Verification items for the finished model (mm, model axes). Round coordinates to 2 decimals unless told otherwise and drop trailing zeros. Loops run counter-clockwise (first coordinate to the right, second up) from the corner with the lowest first, then second, coordinate; pieces in that order, holes last. Notation, with made-up numbers: M -37,60 L -18,60 A29 ccw -18,83 Z; hole C -37,51.25 d2. An arc over 180 degrees is marked long. Answer as CSV lines item,"result".
```python
from build123d import *

# Parameters (mm, degrees)
F0_W     = 53.34
F0_H     = 53.34
F1_DEPTH = 27.78125
F3_R     = 6.35
F4_DEPTH = 38.1
F5_SIZE  = 16.4973
F6_SIZE  = 16.51


with BuildPart() as f1:
    # F0 (on Front) → F1 (new body)
    with BuildSketch(Plane.XZ):
        Rectangle(F0_W, F0_H)
        with BuildLine():
            ThreePointArc((0, 25.4), (17.9605122421, 17.9605122421), (25.4, 0))
            ThreePointArc((25.4, 0), (17.9605122421, -17.9605122421), (0, -25.4))
            ThreePointArc((0, -25.4), (-25.4, 0), (0, 25.4))
        make_face(mode=Mode.SUBTRACT)
        with BuildLine():
            Line((0, -25.4), (0, 25.4))
            ThreePointArc((0, 25.4), (-25.4, 0), (0, -25.4))
        make_face()
        with BuildLine():
            ThreePointArc((0, -25.4), (17.9605122421, -17.9605122421), (25.4, 0))
            ThreePointArc((25.4, 0), (17.9605122421, 17.9605122421), (0, 25.4))
            Line((0, 25.4), (0, -25.4))
        make_face()
    extrude(amount=-F1_DEPTH)

    # F0 (on Front) → F2 (revolve, cut)
    with BuildSketch(Plane.XZ):
        with BuildLine():
            ThreePointArc((0, -25.4), (17.9605122421, -17.9605122421), (25.4, 0))
            ThreePointArc((25.4, 0), (17.9605122421, 17.9605122421), (0, 25.4))
            Line((0, 25.4), (0, -25.4))
        make_face()
    revolve(axis=Axis((0, 0, 0), (0, 0, 1)), mode=Mode.SUBTRACT)

    # F3 (on Top) → F4 (cut)
    with BuildSketch(Plane.XY):
        Circle(F3_R)
    extrude(amount=-F4_DEPTH, mode=Mode.SUBTRACT)

    # F5
    f5_edges = [f1.edges().sort_by_distance(p)[0] for p in [
        (26.67, 27.78125, 0),
    ]]
    chamfer(f5_edges, length=F5_SIZE)

    # F6
    f6_edges = [f1.edges().sort_by_distance(p)[0] for p in [
        (-26.67, 27.78125, 0),
    ]]
    chamfer(f6_edges, length=F6_SIZE)


solid = f1.part
```
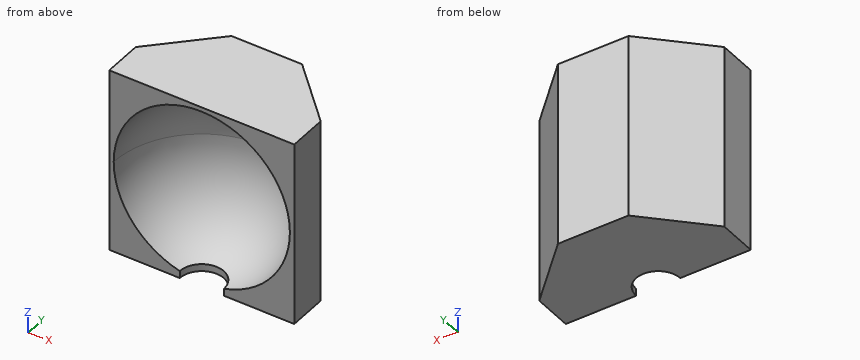
1) Go/stop test with a flat-tipped pin: pin 1 (8 mm diameter, centred on y = 22, z = 10.5, fed in from +X). Record where the tip stops, or that it passes through.
Here are the results:
pin 1,"stops at x = 19.95"
2) Section check B-B (y = 21). Record the cut outline in (x, z), plus the area to 3 significant figures.
Here are the results:
outline,"M -16.94,-26.67 L 16.95,-26.67 L 16.95,26.67 L -16.94,26.67 Z; hole C 0,0 d28.58"
area,"1,170 mm^2"
3) Section check D-D (y = 3.75). Record the cut outline in (x, z), plus the area to 3 significant figures.
Here are the results:
outline,"M -26.67,-26.67 L -5.12,-26.67 L -5.12,-24.59 A25.12 cw long 5.12,-24.59 L 5.12,-26.67 L 26.67,-26.67 L 26.67,26.67 L -26.67,26.67 Z"
area,"845 mm^2"
4) Section check C-C (z = 17). Record the cut outline in (x, y), plus the area to 3 significant figures.
Here are the results:
outline,"M -26.67,0 L -18.87,0 A18.87 cw 18.87,0 L 26.67,0 L 26.67,11.28 L 10.17,27.78 L -10.16,27.78 L -26.67,11.27 Z"
area,"650 mm^2"
5) Material ranges on probe 1 along X at (y, z) = (16.25, 2); probe 2 along Z at (x, y) = (-1, 10.75); probe 3 along X at (y, z) = (17.25, 3), recorded low to high.
Here are the results:
probe 1,"x = -21.69 to -19.42, 19.42 to 21.7"
probe 2,"z = -26.67 to -22.99, 22.99 to 26.67"
probe 3,"x = -20.69 to -18.4, 18.4 to 20.7"
6) Section check A-A (x = 0). Record the cut outline in (y, z).
Here are the results:
outline,"M 0,25.4 A25.4 cw 6.35,-24.59 L 6.35,-26.67 L 27.78,-26.67 L 27.78,26.67 L 0,26.67 Z"
